Part model, mm, in its own coordinate system. Face numbers are marked on the shaded views. A direction names the side the tool comes from. Coordinates: 2 decimals unless noted, no trailing zeros. Loops run counter-clockwise (first coordinate to the right, second up) from the corner with the lowest first, then second, coordinate; pieces in that order, holes last.
```python
from build123d import *

# Parameters (mm, degrees)
BOSS_EXTRU_1_DEPTH      = 2
ESQUISSE2_R             = 1.5
ENL_V_MAT_EXTRU_1_DEPTH = 2


with BuildPart() as part:
    # Esquisse1 → Boss.-Extru.1 (new body)
    with BuildSketch(Plane.XY):
        with BuildLine():
            ThreePointArc((-30.69312299, 5.146506838), (-29.724192295, 5.477574873), (-28.703807813, 5.392438272))
            Line((-28.703807813, 5.392438272), (-23.228481357, 3.761582946))
            Line((-23.228481357, 3.761582946), (-16.714786598, 7.626279325))
            Line((-16.714786598, 7.626279325), (-15.522036632, 13.213428546))
            ThreePointArc((-15.522036632, 13.213428546), (-15.107728814, 14.149794802), (-14.352789293, 14.841531062))
            Line((-14.352789293, 14.841531062), (-30.69312299, 5.146506838))
        make_face()
        with BuildLine():
            Line((-23.228481357, 3.761582946), (-28.703807813, 5.392438272))
            ThreePointArc((-28.703807813, 5.392438272), (-29.724192295, 5.477574873), (-30.69312299, 5.146506838))
            ThreePointArc((-30.69312299, 5.146506838), (-31.89857385, 2.689732543), (-30.131116002, 0.60048759))
            ThreePointArc((-30.131116002, 0.60048759), (-29.11073152, 0.515350989), (-28.141800825, 0.846419024))
            Line((-28.141800825, 0.846419024), (-23.228481357, 3.761582946))
        make_face()
        with BuildLine():
            ThreePointArc((-28.141800825, 0.846419024), (-29.11073152, 0.515350989), (-30.131116002, 0.60048759))
            Line((-30.131116002, 0.60048759), (-16.898324022, -3.333026779))
            ThreePointArc((-16.898324022, -3.333026779), (-18.198183706, -2.190793179), (-18.44490842, -0.478058609))
            Line((-18.44490842, -0.478058609), (-17.879921595, 2.168485758))
            Line((-17.879921595, 2.168485758), (-23.228481357, 3.761582946))
            Line((-23.228481357, 3.761582946), (-28.141800825, 0.846419024))
        make_face()
        with BuildLine():
            Line((-15.286345905, 1.395975341), (-17.879921595, 2.168485758))
            Line((-17.879921595, 2.168485758), (-18.44490842, -0.478058609))
            ThreePointArc((-18.44490842, -0.478058609), (-18.198183706, -2.190793179), (-16.898324022, -3.333026779))
            Line((-16.898324022, -3.333026779), (-16.521941391, -3.44490842))
            ThreePointArc((-16.521941391, -3.44490842), (-14.640256973, -3.09787962), (-13.55509158, -1.521941391))
            ThreePointArc((-13.55509158, -1.521941391), (-13.849956093, 0.275661082), (-15.286345905, 1.395975341))
        make_face()
        with BuildLine():
            Line((-16.714786598, 7.626279325), (-17.879921595, 2.168485758))
            Line((-17.879921595, 2.168485758), (-15.286345905, 1.395975341))
            ThreePointArc((-15.286345905, 1.395975341), (-13.849956093, 0.275661082), (-13.55509158, -1.521941391))
            Line((-13.55509158, -1.521941391), (-10.632219791, 12.169545764))
            ThreePointArc((-10.632219791, 12.169545764), (-11.046527609, 11.233179508), (-11.801467129, 10.541443247))
            Line((-11.801467129, 10.541443247), (-16.714786598, 7.626279325))
        make_face()
        with BuildLine():
            Line((-15.522036632, 13.213428546), (-16.714786598, 7.626279325))
            Line((-16.714786598, 7.626279325), (-11.801467129, 10.541443247))
            ThreePointArc((-11.801467129, 10.541443247), (-11.046527609, 11.233179508), (-10.632219791, 12.169545764))
            ThreePointArc((-10.632219791, 12.169545764), (-11.618820564, 14.722087757), (-14.352789293, 14.841531062))
            ThreePointArc((-14.352789293, 14.841531062), (-15.107728814, 14.149794802), (-15.522036632, 13.213428546))
        make_face()
    extrude(amount=-BOSS_EXTRU_1_DEPTH)

    # Esquisse2 → Enlèv. mat.-Extru.1 (cut)
    with BuildSketch(Plane.XY):
        with Locations((-29.417461908, 2.996462931)):
            Circle(ESQUISSE2_R)
        with Locations((-16, -1)):
            Circle(ESQUISSE2_R)
        with Locations((-13.077128211, 12.691487155)):
            Circle(ESQUISSE2_R)
    extrude(amount=-ENL_V_MAT_EXTRU_1_DEPTH, mode=Mode.SUBTRACT)


solid = part.part
```
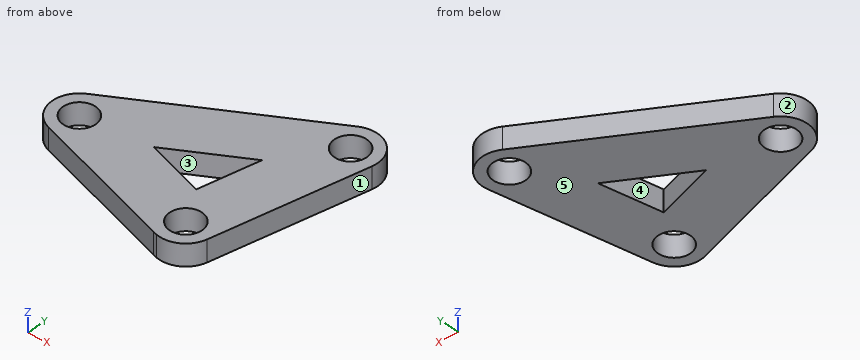
Q1. Saw through at A-A (y = -1). List the corners of the cut face in (x, z).
Q2. Probe line 1 (X direction, y = 4, z = -0.85); line 2 (X direction, y = 6, z = -0.8); line 3 (Y direction, x = -16, z = -1.5). List the from-to ranges inside material, lowest first.
Q3. Mould opens along Y. For the marked faces 1, 2 and 3 say: released by +Y, released by -Y, zero draft, split by the parting line, or undercut.
Q4. Tool access for the marked faces 4 and 5: list every direction of +Z, -Z, +X, -X, +Y, -Y with a clear straight run to the whole face (end or side of a thin tool).
Q5. Saw through at C-C (z = -0.25). List the corners of the cut face in (x, y).
Q6. Saw through at D-D (x = -24.25). List the corners of the cut face in (y, z).
Q7. Drop flat-ended pins along their axis: P1, Ø1, axis at x = -17.5, z = -1.5, coming from the -Y side; P2, Ø1, axis at x = -29, z = -1.5, coming from the -Y side. Give the stop position or say it passes through.
Q8. Saw through at B-B (x = -20.75). List the corners of the cut face in (y, z).
Checked values:
1. outline: (-24.75, -2) - (-17.5, -2) - (-17.5, 0) - (-24.75, 0) - close; (-14.5, -2) - (-13.44, -2) - (-13.44, 0) - (-14.5, 0) - close
2. line 1: x = -31.71 to -30.53, -28.3 to -22.83, -17.49 to -12.38
2. line 2: x = -29.25 to -19.46, -17.06 to -11.95
2. line 3: y = -3.5 to -2.5, 0.5 to 13.86
3. face 1: released by -Y
3. face 2: split by the parting line
3. face 3: undercut
4. face 4: +Z, -Z
4. face 5: -Z, +X, -X, +Y, -Y
5. outline: (-30.69, 5.15) arc R2.5 ccw to (-30.13, 0.6) - (-16.52, -3.44) arc R2.5 ccw to (-13.56, -1.52) - (-10.63, 12.17) arc R2.5 ccw to (-14.35, 14.84) - close; hole circle Ø3 at (-29.42, 3); hole (-23.23, 3.76) - (-17.88, 2.17) - (-16.71, 7.63) - close; hole circle Ø3 at (-16, -1); hole circle Ø3 at (-13.08, 12.69)
6. outline: (-1.15, -2) - (8.97, -2) - (8.97, 0) - (-1.15, 0) - close
7. P1: stops at y = -3.3
7. P2: stops at y = 0.12
8. outline: (-2.19, -2) - (3.02, -2) - (3.02, 0) - (-2.19, 0) - close; (5.23, -2) - (11.05, -2) - (11.05, 0) - (5.23, 0) - close
